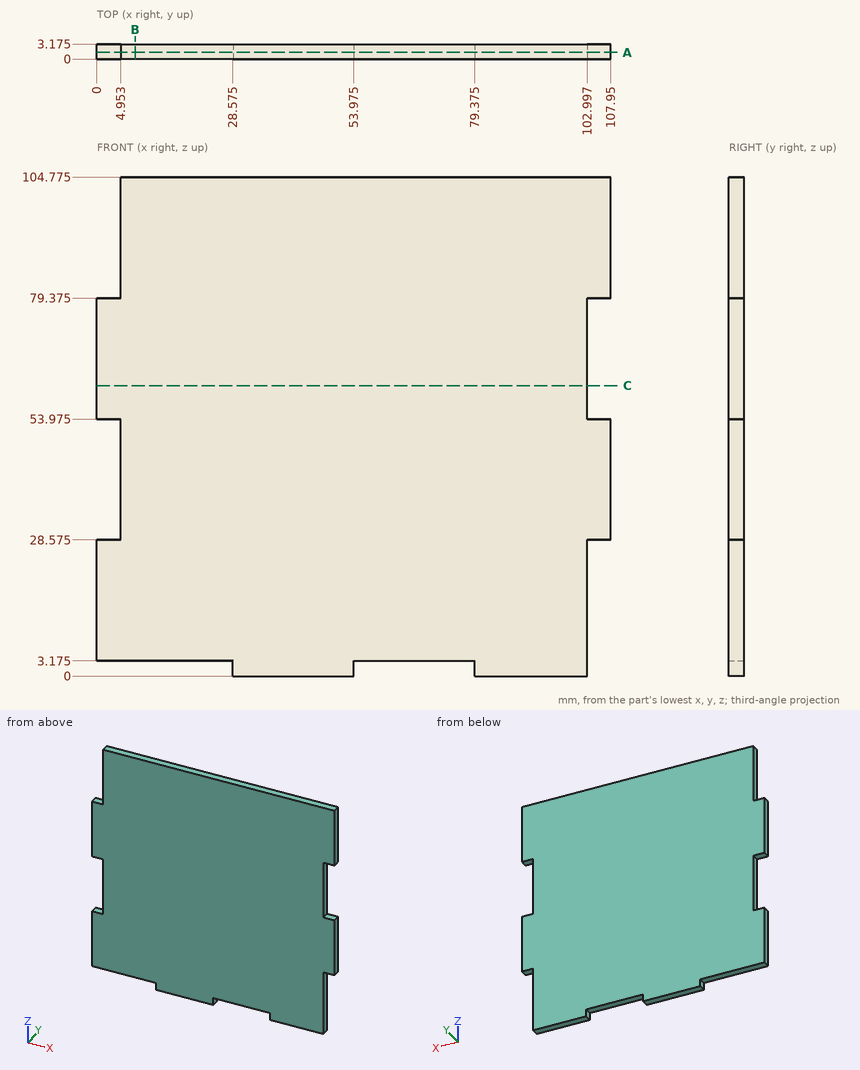
The figure shows three views and two pictorial views of one solid part (mm, origin at its lowest corner). Answer the questions. Give positions to 0.01 mm unless a question says otherwise; leave off trailing zeros. Loops run counter-clockwise (first coordinate to the right, second up) from the corner with the lowest first, then second, coordinate; pieces in that order, holes last. Notation, with made-up numbers: (83.25, 88) -> (102.25, 88) arc R19 cw to (102.25, 105) -> close; hole circle Ø2 at (76, 45.5). An arc over 180 degrees is marked (long way). Put each result on its own line as item: value. Start each with the question number.
Item 1: Find the intervals of material crossed by L1, parallel to X at y = 2.9, z = 91; L2, parallel to Z at x = 76.5, y = 0.5 (3 decimals); L3, parallel to X at y = 2.25, z = 4, in increasing order. Write a range as [from, to].
Item 2: Each of these flat-tipped pins is pushed along its axis until it touches: P1, Ø1.5, axis at x = 36, z = 85, coming from the -Y side; P2, Ø1, axis at x = 105.5, y = 1.5, coming from the -Z side (3 decimals); P3, Ø1.6, axis at y = 2, z = 1, coming from the +X side; P4, Ø1.6, axis at x = 3, y = 1, coming from the +Z side (3 decimals). Where does it stop, or does it pass through?
Item 3: The part is cut by section B-B (x = 8). Give the vertices of the cut face in (y, z) (3 decimals).
Item 4: The part is cut by section C-C (z = 61). Give the vertices of the cut face in (x, y) (3 decimals), then the cut area to 3 significant figures.
Item 5: The part is cut by section A-A (y = 1.4). Give the vertices of the cut face in (x, z) (3 decimals), then the cut area to 3 significant figures.
Answers below:
1. L1: [4.95, 107.95]
1. L2: [3.175, 104.775]
1. L3: [0, 103]
2. P1: y = 0
2. P2: z = 28.575
2. P3: x = 103
2. P4: z = 79.375
3. outline: (0, 3.175) -> (3.175, 3.175) -> (3.175, 104.775) -> (0, 104.775) -> close
4. outline: (0, 0) -> (102.997, 0) -> (102.997, 3.175) -> (0, 3.175) -> close
4. area: 327 mm2
5. outline: (0, 3.175) -> (28.575, 3.175) -> (28.575, 0) -> (53.975, 0) -> (53.975, 3.175) -> (79.375, 3.175) -> (79.375, 0) -> (102.997, 0) -> (102.997, 28.575) -> (107.95, 28.575) -> (107.95, 53.975) -> (102.997, 53.975) -> (102.997, 79.375) -> (107.95, 79.375) -> (107.95, 104.775) -> (4.953, 104.775) -> (4.953, 79.375) -> (0, 79.375) -> (0, 53.975) -> (4.953, 53.975) -> (4.953, 28.575) -> (0, 28.575) -> close
5. area: 10,600 mm2
